Can you work these out from the model? Positions are in its coordinate system, mm. A direction names the side the tool comes from. Round coordinates to 2 decimals unless told otherwise and drop trailing zeros. Write each loop counter-clockwise with the first axis right and the second up, starting at its lowest first coordinate (ties: lowest second). Pieces come first, ordered by that corner, then holes. Notation, with made-up numbers: (45, 39.25) -> (65, 39.25) arc R22 ccw to (65, 50.25) -> close; hole circle Ø6 at (89, 26). An arc over 180 degrees is marked (long way). Use CSV: the item, a comma, the result in double quotes.
Autodesk Inventor part; units mm, degrees
ref_plane "YZ Plane" through (0, 0, 0) normal (1, 0, 0) x (0, 1, 0)
ref_plane "XZ Plane" through (0, 0, 0) normal (0, 1, 0) x (-1, 0, 0)
ref_plane "XY Plane" through (0, 0, 0) normal (0, 0, 1) x (1, 0, 0)
sketch "Sketch1" plane through (0, 0, 0) normal (0, 1, 0) x (-1, 0, 0)
  line L0 (0, -37.5) -> (0, 0)
  line L1 (0, 0) -> (-74.5, 0)
  line L2 (-74.5, 0) -> (-74.5, -20)
  line L3 (-74.5, -20) -> (-15, -37.5)
  line L4 (-15, -37.5) -> (0, -37.5)
  dimension "d0" = 37.5
  dimension "d1" = 74.5
  dimension "d2" = 20
  dimension "d3" = 15
extrude "Extrusion1" add sketch "Sketch1" along normal blind 6.5
sketch "Sketch2" plane through (0, 0, 0) normal (0, -1, 0) x (1, 0, 0)
  line L0 (0, 0) -> (0, -37.5)
  line L1 (0, -37.5) -> (15, -37.5)
  line L2 (16.3, -23.5) -> (16.3, -28)
  line L3 (0, -28) -> (0, -23.5)
  line L4 (5, -21) -> (12.3, -21)
  line L5 (12.3, -30.5) -> (5, -30.5)
  line L6 (0, -23.5) -> (5, -23.5)
  line L7 (12.3, -23.5) -> (16.3, -23.5)
  line L8 (16.3, -28) -> (12.3, -28)
  line L9 (5, -28) -> (0, -28)
  line L10 (5, -30.5) -> (5, -28)
  line L11 (5, -23.5) -> (5, -21)
  line L12 (12.3, -21) -> (12.3, -23.5)
  line L13 (12.3, -28) -> (12.3, -30.5)
  point P0 (16.3, -25.75)
  dimension "d6" = 4.5
  dimension "d7" = 2.5
  dimension "d8" = 5
  dimension "d9" = 7.3
  dimension "d10" = 4
  dimension "d12" = 14
extrude "Extrusion2" cut sketch "Sketch2" against normal through all
sketch "Sketch3" plane through (0, 0, 0) normal (0, -1, 0) x (1, 0, 0)
  line L0 (74.5, -20) -> (74.5, 0)
  line L1 (74.5, 0) -> (0, 0)
  line L2 (66.5, 0) -> (58.5, 0)
  line L3 (58.5, 0) -> (58.5, 4.5)
  line L4 (60.5, 6.5) -> (64.5, 6.5)
  line L5 (66.5, 4.5) -> (66.5, 0)
  arc A0 (60.5, 6.5) -> (58.5, 4.5) centre (60.5, 4.5) ccw
  arc A1 (66.5, 4.5) -> (64.5, 6.5) centre (64.5, 4.5) ccw
  dimension "d15" = 2
  dimension "d16" = 8
  dimension "d17" = 6.5
  dimension "d18" = 8
extrude "Extrusion3" add sketch "Sketch3" against normal blind 6.5
sketch "Sketch4" plane through (0, 0, 0) normal (0, -1, 0) x (1, 0, 0)
  line L0 (58.5, 4.5) -> (58.5, 0)
  line L1 (58.5, 0) -> (0, 0)
  line L2 (36.25, 0) -> (40.75, 0)
  line L3 (40.75, -16.3) -> (36.25, -16.3)
  line L4 (43.25, -5) -> (43.25, -12.3)
  line L5 (33.75, -12.3) -> (33.75, -5)
  line L6 (33.75, -5) -> (36.25, -5)
  line L7 (40.75, -5) -> (43.25, -5)
  line L8 (43.25, -12.3) -> (40.75, -12.3)
  line L9 (36.25, -12.3) -> (33.75, -12.3)
  line L10 (36.25, -16.3) -> (36.25, -12.3)
  line L11 (36.25, -5) -> (36.25, 0)
  line L12 (40.75, 0) -> (40.75, -5)
  line L13 (40.75, -12.3) -> (40.75, -16.3)
  point P0 (38.5, -16.3)
  dimension "d21" = 4.5
  dimension "d22" = 2.5
  dimension "d23" = 5
  dimension "d24" = 4
  dimension "d25" = 7.3
  dimension "d26" = 20
extrude "Extrusion4" cut sketch "Sketch4" against normal through all
sketch "Sketch6" plane through (0, 6.5, 0) normal (0, 1, 0) x (1, 0, 0)
  line L0 (40.75, 0) -> (58.5, 0)
  line L1 (74.5, 0) -> (74.5, 20)
  line L2 (74.5, 20) -> (15, 37.5)
  arc A0 (51.3532, 26.8079) -> (60.8316, 24.0201) centre (54.5, 20) ccw
  circle A1 centre (54.5, 20) radius 4 construction
  line L3 (51.3532, 26.8079) -> (60.8316, 24.0201)
  dimension "d34" = 15
  dimension "d35" = 8
  dimension "d36" = 20
  dimension "d37" = 20
extrude "Extrusion6" cut sketch "Sketch6" against normal through all
chamfer "Chamfer1" distance 1 angle 45 2 edges at (51.3532, 3.25, -26.8079) (60.8316, 3.25, -24.0201)
chamfer "Chamfer2" distance 2 angle 45 1 edges at (74.5, 3.25, -20)
chamfer "Chamfer3" distance 6 angle 45 1 edges at (0, 3.25, 0)
sketch "Sketch7" plane through (0, 6.5, 0) normal (0, 1, 0) x (1, 0, 0)
  line L0 (66.5, 0) -> (74.5, 0)
  line L1 (74.5, 0) -> (74.5, 18)
  circle A0 centre (66.5, 12) radius 2.25
  point P0 (0, 0)
  dimension "d49" = 4.5
  dimension "d50" = 8
  dimension "d51" = 12
extrude "Extrusion7" cut sketch "Sketch7" against normal through all
properties part number "x_carryage_brace_bottom" material "Plywood, Finish"
Q1. On a 3-axis mill with a long thin cutter (end or side, diameter ignored), from which of +Z, -Z, +X, -X, +Y, -Y can I reach the whole of each face in a straight line? I mean faces 1 (the face through (14, 3, -28)), 2 (the face through (12.3, 3, -29)), 3 (the face through (70, 3, 0)). Say none if no direction works.
Resolved:
face 1,"-X, +Y, -Y"
face 2,"+Y, -Y"
face 3,"+Z, +X, +Y, -Y"
Q2. Suppose I cut it at A-A (z = -3). Write out the boundary of the cut face in (x, y), and give its area (4 significant figures).
Resolved:
outline,"(3, 0) -> (36.25, 0) -> (36.25, 6.5) -> (3, 6.5) -> close; (40.75, 0) -> (74.5, 0) -> (74.5, 6.5) -> (40.75, 6.5) -> close"
area,"435.5 mm^2"
Q3. Will these pins go through, and if not, where does the flat tip stop? P1, Ø2, axis at x = 8, y = 3.5, coming from the +Z side; P2, Ø3, axis at x = 35.5, y = 4, coming from the -Z side; P3, Ø3.5, axis at y = 3, z = 1.5, coming from the -X side.
Resolved:
P1,"stops at z = 0"
P2,"stops at z = -31.91"
P3,"stops at x = 5.75"
Q4. If we mould it in two halves opening along Z, with no side actions, what happens to faces 4 (the face through (14, 3, -23.5)), 5 (the face through (3, 3, -3)), 6 (the face through (0, 3, -33))? For each: released by +Z, released by -Z, zero draft, split by the parting line, or undercut.
Resolved:
face 4,"undercut"
face 5,"released by +Z"
face 6,"zero draft"
Q5. Suppose I cut it at B-B (x = 20). Write out the boundary of the cut face in (y, z), and give its area (3 significant figures).
Resolved:
outline,"(0, -36.03) -> (6.5, -36.03) -> (6.5, 0) -> (0, 0) -> close"
area,"234 mm^2"
Q6. Suppose I cut it at C-C (x = 44). Write out the boundary of the cut face in (y, z).
Resolved:
outline,"(0, -28.97) -> (6.5, -28.97) -> (6.5, 0) -> (0, 0) -> close"
Q7. Please list where these lines run through material, in increasing order: probe 1 along X at (y, z) = (3.25, -12); probe 2 along X at (y, z) = (2.75, -6); probe 3 along Z at (x, y) = (11, 5).
Resolved:
probe 1,"x = 0 to 33.75, 43.25 to 64.25, 68.75 to 74.5"
probe 2,"x = 0 to 33.75, 43.25 to 74.5"
probe 3,"z = -37.5 to -30.5, -21 to 0"
